Design review of the part built by this model. Coordinates are the model's own, in mm. Face numbers are marked on the shaded views. A direction names the side the tool comes from. Coordinates: 2 decimals unless noted, no trailing zeros. Loops run counter-clockwise (first coordinate to the right, second up) from the corner with the lowest first, then second, coordinate; pieces in that order, holes last. Notation, with made-up numbers: (3, 3.5) - (53, 3.5) arc R17 cw to (53, 24.5) - close; hole circle Ø6 at (-5.75, -28). An arc over 180 degrees is marked (long way). Use one line per item in the form item = value. Start each with the question number.
(1) Clearance check with flat-ended pins moving along their axes: pin 1 Ø1 at (y, z) = (5.5, 12.5) entering from +X; pin 2 Ø5 at (x, y) = (12.73, 12.73) entering from +Z; pin 3 Ø3 at (y, z) = (0, 4) entering from -X; pin 4 Ø4.5 at (x, z) = (1, 7.5) entering from +Y. State where each tip first meets the part, or that it passes through.
(2) Add section C-C (x = 12.5). State the section outline as (y, z) points, plus the area to 3 significant figures.
(3) The part is to be moulded in two halves that separate along Y. For the marked faces 1, 2 and 3, say which applies: pulls with the +Y half, pulls with the -Y half, needs draft (parallel to the pull), parting line crosses it, or undercut.
(4) Tool access review of the marked faces 4, 5 and 6: name each direction out of +Z, -Z, +X, -X, +Y, -Y from which nothing blocks a thin tool from reaching the whole face with its end or side.
(5) Add section A-A (x = 0). State the section outline as (y, z) points, plus the area to 3 significant figures.
(6) Add section D-D (z = 4.5). Count the separate pieces of the cut face and the enclosed holes in it, plus the area to 3 significant figures.
(7) Add section B-B (y = 0). State the section outline as (x, z) points.
(8) For L1, parallel to Z at x = 0, y = -5.2; L2, parallel to Y at x = 1.5, z = 3.5; L3, parallel to Y at x = 13.5, z = 3.5, list the stretches that pass through material, from the lowest coordinate up.
```python
from build123d import *

# Parameters (mm, degrees)
SKETCH_1_R          = 2
SKETCH_1_R_2        = 4.05
EXTRUDE_1_DEPTH     = 15.5
FILLET_3_R          = 3
SKETCH_3_R          = 1.5
CUT_EXTRUDE_2_DEPTH = 35.677503091


with BuildPart() as part:
    # ｽｹｯﾁ1 → ﾎﾞｽ - 押し出し1 (new body)
    with BuildSketch(Plane.XY):
        Polygon((-7.727922061, 17.727922061), (-7.727922061, 7.727922061), (7.727922061, 7.727922061), (7.727922061, 17.727922061), (17.727922061, 17.727922061), (17.727922061, 5), (7.727922061, 5), (7.727922061, -5), (17.727922061, -5), (17.727922061, -17.727922061), (7.727922061, -17.727922061), (7.727922061, -7.727922061), (-7.727922061, -7.727922061), (-7.727922061, -17.727922061), (-17.727922061, -17.727922061), (-17.727922061, -5), (-7.727922061, -5), (-7.727922061, 5), (-17.727922061, 5), (-17.727922061, 17.727922061), align=None)
        with Locations((-12.727922061, 12.727922061)):
            Circle(SKETCH_1_R, mode=Mode.SUBTRACT)
        with Locations((12.727922061, 12.727922061)):
            Circle(SKETCH_1_R, mode=Mode.SUBTRACT)
        with Locations((12.727922061, -12.727922061)):
            Circle(SKETCH_1_R, mode=Mode.SUBTRACT)
        with Locations((-12.727922061, -12.727922061)):
            Circle(SKETCH_1_R, mode=Mode.SUBTRACT)
        Circle(SKETCH_1_R_2, mode=Mode.SUBTRACT)
    extrude(amount=EXTRUDE_1_DEPTH)

    # ﾌｨﾚｯﾄ3
    fillet_3_edges = [part.edges().sort_by_distance(p)[0] for p in [
        (-17.727922061, 17.727922061, 7.75),
        (-7.727922061, 17.727922061, 7.75),
        (-7.727922061, 7.727922061, 7.75),
        (7.727922061, 7.727922061, 7.75),
        (7.727922061, 17.727922061, 7.75),
        (17.727922061, 17.727922061, 7.75),
        (17.727922061, 5, 7.75),
        (7.727922061, 5, 7.75),
        (7.727922061, -5, 7.75),
        (17.727922061, -5, 7.75),
        (17.727922061, -17.727922061, 7.75),
        (7.727922061, -17.727922061, 7.75),
        (7.727922061, -7.727922061, 7.75),
        (-7.727922061, -7.727922061, 7.75),
        (-7.727922061, -17.727922061, 7.75),
        (-17.727922061, -17.727922061, 7.75),
        (-17.727922061, -5, 7.75),
        (-7.727922061, -5, 7.75),
        (-7.727922061, 5, 7.75),
        (-17.727922061, 5, 7.75),
    ]]
    fillet(fillet_3_edges, radius=FILLET_3_R)

    # ｽｹｯﾁ3 → ｶｯﾄ - 押し出し2 (cut, through all)
    with BuildSketch(Plane(origin=(0, 7.727922061, 0), x_dir=(1, 0, 0), z_dir=(0, 1, 0))):
        with Locations(Location((0, -4, 0), (0, 0, 270))):
            Circle(SKETCH_3_R)
        with Locations(Location((0, -11.5, 0), (0, 0, 270))):
            Circle(SKETCH_3_R)
    extrude(amount=-CUT_EXTRUDE_2_DEPTH, mode=Mode.SUBTRACT)


solid = part.part
```
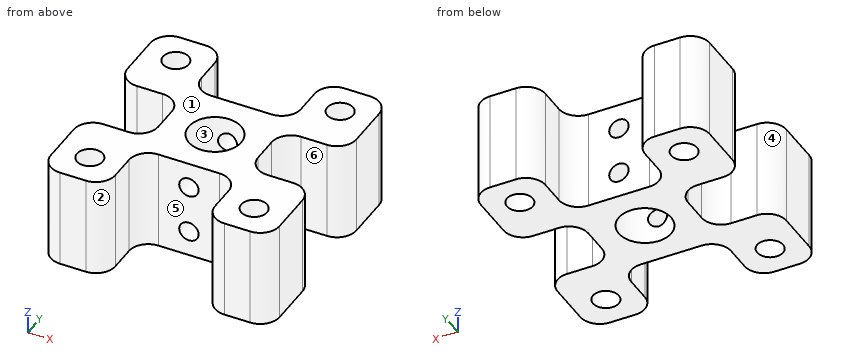
Computed values:
q1.pin_1 = 16.96
q1.pin_2 = 15.5
q1.pin_3 = -7.73
q1.pin_4 = 7.73
q2.outline = (-17.73, 0) - (-14.71, 0) - (-14.71, 15.5) - (-17.73, 15.5) - close; (-10.74, 0) - (-5, 0) - (-5, 15.5) - (-10.74, 15.5) - close; (5, 0) - (10.74, 0) - (10.74, 15.5) - (5, 15.5) - close; (14.71, 0) - (17.73, 0) - (17.73, 15.5) - (14.71, 15.5) - close
q2.area = 271 mm^2
q3.face_1 = needs draft
q3.face_2 = pulls with the -Y half
q3.face_3 = undercut
q4.face_4 = +Z, -Z, -X
q4.face_5 = +Z, -Z, -Y
q4.face_6 = +Z, -Z, +X
q5.outline = (-7.73, 0) - (-4.05, 0) - (-4.05, 2.5) - (-7.73, 2.5) - close; (-7.73, 5.5) - (-4.05, 5.5) - (-4.05, 10) - (-7.73, 10) - close; (-7.73, 13) - (-4.05, 13) - (-4.05, 15.5) - (-7.73, 15.5) - close; (4.05, 0) - (7.73, 0) - (7.73, 2.5) - (4.05, 2.5) - close; (4.05, 5.5) - (7.73, 5.5) - (7.73, 10) - (4.05, 10) - close; (4.05, 13) - (7.73, 13) - (7.73, 15.5) - (4.05, 15.5) - close
q5.area = 69.9 mm^2
q6.separate_pieces = 2
q6.enclosed_holes = 4
q6.area = 617 mm^2
q7.outline = (-7.73, 0) - (-4.05, 0) - (-4.05, 15.5) - (-7.73, 15.5) - close; (4.05, 0) - (7.73, 0) - (7.73, 15.5) - (4.05, 15.5) - close
q8.L1 = 0 to 2.5, 5.5 to 10, 13 to 15.5
q8.L2 = -7.73 to -3.76, 3.76 to 7.73
q8.L3 = -17.73 to -14.57, -10.88 to -5, 5 to 10.88, 14.57 to 17.73
